Build history of the part. All positions in model axes, mm. Face numbers are marked on the shaded views. Round coordinates to 2 decimals unless told otherwise and drop trailing zeros. Write each loop counter-clockwise with the first axis right and the second up, starting at its lowest first coordinate (ties: lowest second). Pieces come first, ordered by that corner, then holes. Notation, with made-up numbers: M 19,-11.75 L 76,-11.75 A28 cw 76,12.25 Z; hole C 1.25,35 d6. An arc over 180 degrees is marked long. Write item = value, one per line.
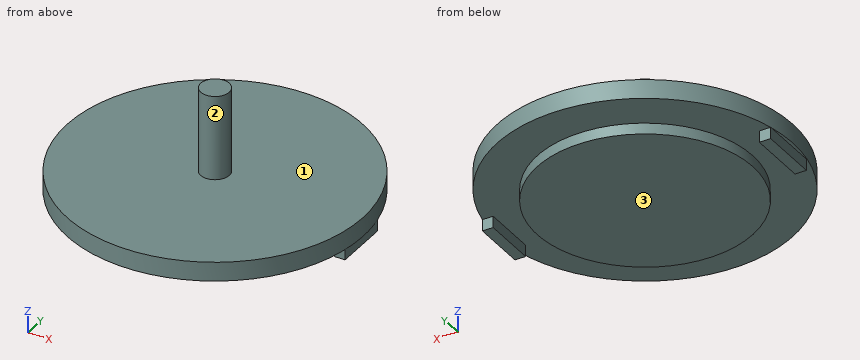
from build123d import *

# Parameters (mm, degrees)
SKETCH1_R           = 77.5
BOSS_EXTRUDE1_DEPTH = 10
SKETCH2_R           = 56.5
BOSS_EXTRUDE2_DEPTH = 5.764188233
SKETCH3_R           = 7.5
BOSS_EXTRUDE3_DEPTH = 60
SKETCH4_W           = 5.635994667
SKETCH4_H           = 28.610379267
SKETCH4_W_2         = 5.979262635
SKETCH4_H_2         = 31.399489247
BOSS_EXTRUDE4_DEPTH = 6


with BuildPart() as part:
    # Sketch1 → Boss-Extrude1 (new body)
    with BuildSketch(Plane.XY):
        Circle(SKETCH1_R)
    extrude(amount=BOSS_EXTRUDE1_DEPTH)

    # Sketch2 → Boss-Extrude2 (add)
    with BuildSketch(Plane(origin=(0, 0, 0), x_dir=(-1, 0, 0), z_dir=(0, 0, -1))):
        Circle(SKETCH2_R)
    extrude(amount=BOSS_EXTRUDE2_DEPTH)

    # Sketch3 → Boss-Extrude3 (add)
    with BuildSketch(Plane(origin=(0, 0, -5.764188233), x_dir=(-1, 0, 0), z_dir=(0, 0, -1))):
        Circle(SKETCH3_R)
    extrude(amount=-BOSS_EXTRUDE3_DEPTH)

    # Sketch4 → Boss-Extrude4 (add)
    with BuildSketch(Plane(origin=(0, 0, 0), x_dir=(-1, 0, 0), z_dir=(0, 0, -1))):
        with Locations((-73.064647, 1.445184616)):
            Rectangle(SKETCH4_W, SKETCH4_H)
        with Locations((72.742981652, 0.756905489)):
            Rectangle(SKETCH4_W_2, SKETCH4_H_2)
    extrude(amount=BOSS_EXTRUDE4_DEPTH)


solid = part.part
1. Probe probe 1 along X at (y, z) = (1.5, -1); probe 2 along Z at (x, y) = (39, -51); probe 3 along Z at (x, y) = (14, -1.5). List the from-to ranges inside material, lowest first.
Responses:
probe_1 = -75.73 to -69.75, -56.48 to 56.48, 70.25 to 75.88
probe_2 = 0 to 10
probe_3 = -5.76 to 10
2. Flat gauge pins, fed straight in: pin 1 (1.8 mm diameter, centred on y = 2.5, z = -3, fed in from +X); pin 2 (1.8 mm diameter, centred on y = 7, z = -4, fed in from -X); pin 3 (12 mm diameter, centred on x = -52, y = 46, fed in from +Z). Where does each tip first touch, or does it go through?
Responses:
pin_1 = 75.88
pin_2 = -75.73
pin_3 = 10
3. Band-saw the part on B-B (x = 0). List the corners of the cut face in (y, z).
Responses:
outline = M -77.5,0 L -56.5,0 L -56.5,-5.76 L 56.5,-5.76 L 56.5,0 L 77.5,0 L 77.5,10 L 7.5,10 L 7.5,54.24 L -7.5,54.24 L -7.5,10 L -77.5,10 Z
4. Band-saw the part on A-A (y = 0). List the corners of the cut face in (x, z).
Responses:
outline = M -77.5,0 L -75.73,0 L -75.73,-6 L -69.75,-6 L -69.75,0 L -56.5,0 L -56.5,-5.76 L 56.5,-5.76 L 56.5,0 L 70.25,0 L 70.25,-6 L 75.88,-6 L 75.88,0 L 77.5,0 L 77.5,10 L 7.5,10 L 7.5,54.24 L -7.5,54.24 L -7.5,10 L -77.5,10 Z
5. Band-saw the part on C-C (z = 16). List the corners of the cut face in (x, y), plus the area to 3 significant figures.
Responses:
outline = C 0,0 d15
area = 177 mm²
6. Mould opens along X. For the marked faces 1, 2 and 3 say: pulls with the +X half, pulls with the -X half, needs draft (parallel to the pull), parting line crosses it, or undercut.
Responses:
face_1 = needs draft
face_2 = parting line crosses it
face_3 = undercut
7. Band-saw the part on D-D (x = -51). List the corners of the cut face in (y, z).
Responses:
outline = M -58.35,0 L -24.32,0 L -24.32,-5.76 L 24.32,-5.76 L 24.32,0 L 58.35,0 L 58.35,10 L -58.35,10 Z
